Geometry: final body of the model. Coordinates: model frame, mm. Give positions to 0.01 mm unless a question says otherwise; leave off trailing zeros. Loops run counter-clockwise (first coordinate to the right, second up) from the corner with the lowest first, then second, coordinate; pieces in that order, holes last. Notation, with made-up numbers: (27.5, 70.5) - (37.5, 70.5) arc R24 ccw to (37.5, 108.5) - close; hole circle Ø5 at (7, 41). An arc over 180 degrees is marked (long way). Use one line per item in the form item = value.
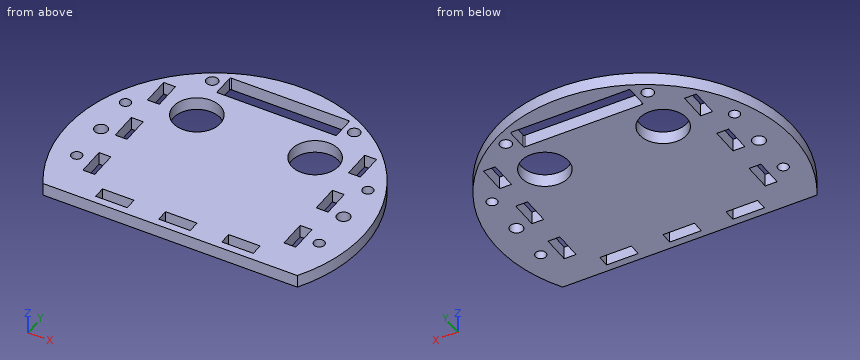
```python
from build123d import *

# Parameters (mm, degrees)
SKETCH1_R           = 2.25
SKETCH1_R_2         = 2.75
SKETCH1_R_3         = 2.5
SKETCH1_R_4         = 10
SKETCH1_W           = 13.333333333
SKETCH1_H           = 4.9958
SKETCH1_W_2         = 4.9958
SKETCH1_H_2         = 11.818181818
SKETCH1_H_3         = 11.818181819
SKETCH1_W_3         = 13.333333334
BOSS_EXTRUDE1_DEPTH = 5.4356


with BuildPart() as part:
    # Sketch1 → Boss-Extrude1 (new body)
    with BuildSketch(Plane.XY):
        with BuildLine():
            Line((-53.750203106, -32.862070326), (53.750203106, -32.862070326))
            ThreePointArc((53.750203106, -32.862070326), (0, 63), (-53.750203106, -32.862070326))
        make_face()
        with Locations((51.25, 23.184046239)):
            Circle(SKETCH1_R, mode=Mode.SUBTRACT)
        with Locations((51.25, -12.496398734)):
            Circle(SKETCH1_R, mode=Mode.SUBTRACT)
        with Locations((-51.25, -12.496398734)):
            Circle(SKETCH1_R, mode=Mode.SUBTRACT)
        with Locations((-51.25, 23.184046239)):
            Circle(SKETCH1_R, mode=Mode.SUBTRACT)
        with Locations((-51.25, 5.343823752)):
            Circle(SKETCH1_R_2, mode=Mode.SUBTRACT)
        with Locations((51.25, 5.343823752)):
            Circle(SKETCH1_R_2, mode=Mode.SUBTRACT)
        with Locations((-30.011103704, 49.928449687)):
            Circle(SKETCH1_R_3, mode=Mode.SUBTRACT)
        with Locations((30.011103704, 49.928449687)):
            Circle(SKETCH1_R_3, mode=Mode.SUBTRACT)
        with Locations((-25, 29.983449687)):
            Circle(SKETCH1_R_4, mode=Mode.SUBTRACT)
        with Locations((25, 29.983449687)):
            Circle(SKETCH1_R_4, mode=Mode.SUBTRACT)
        with BuildLine():
            Line((-24.765, 54.873449687), (24.765, 54.873449687))
            ThreePointArc((24.765, 54.873449687), (25.118553391, 54.727003078), (25.265, 54.373449687))
            Line((25.265, 54.373449687), (25.265, 45.483449687))
            ThreePointArc((25.265, 45.483449687), (25.118553391, 45.129896297), (24.765, 44.983449687))
            Line((24.765, 44.983449687), (-24.765, 44.983449687))
            ThreePointArc((-24.765, 44.983449687), (-25.118553391, 45.129896297), (-25.265, 45.483449687))
            Line((-25.265, 45.483449687), (-25.265, 54.373449687))
            ThreePointArc((-25.265, 54.373449687), (-25.118553391, 54.727003078), (-24.765, 54.873449687))
        make_face(mode=Mode.SUBTRACT)
        with Locations((-26.666666666, -27.189170326)):
            Rectangle(SKETCH1_W, SKETCH1_H, mode=Mode.SUBTRACT)
        with Locations((42.4979, 34.399638765)):
            Rectangle(SKETCH1_W_2, SKETCH1_H_2, mode=Mode.SUBTRACT)
        with Locations((42.4979, 10.763275129)):
            Rectangle(SKETCH1_W_2, SKETCH1_H_3, mode=Mode.SUBTRACT)
        with Locations((-42.4979, 34.399638765)):
            Rectangle(SKETCH1_W_2, SKETCH1_H_2, mode=Mode.SUBTRACT)
        with Locations((-42.4979, 10.763275129)):
            Rectangle(SKETCH1_W_2, SKETCH1_H_3, mode=Mode.SUBTRACT)
        with Locations((-42.4979, -12.873088508)):
            Rectangle(SKETCH1_W_2, SKETCH1_H_2, mode=Mode.SUBTRACT)
        with Locations((42.4979, -12.873088508)):
            Rectangle(SKETCH1_W_2, SKETCH1_H_2, mode=Mode.SUBTRACT)
        with Locations((0, -27.189170326)):
            Rectangle(SKETCH1_W_3, SKETCH1_H, mode=Mode.SUBTRACT)
        with Locations((26.666666666, -27.189170326)):
            Rectangle(SKETCH1_W, SKETCH1_H, mode=Mode.SUBTRACT)
    extrude(amount=BOSS_EXTRUDE1_DEPTH)


solid = part.part
```
(1) Cut plane C-C (y = 13). Return the cut outline in (x, z), plus the area to 3 significant figures.
Solution:
outline = (-61.64, 0) - (-45, 0) - (-45, 5.44) - (-61.64, 5.44) - close; (-40, 0) - (40, 0) - (40, 5.44) - (-40, 5.44) - close; (45, 0) - (61.64, 0) - (61.64, 5.44) - (45, 5.44) - close
area = 616 mm2
(2) Material intervals for L1, parallel to Y at x = -51.25, z = 2.6; L2, parallel to Y at x = -5.5, z = 2.1; L3, parallel to Y at x = -25, z = 3.15, sorted ascending. Write a range as from..to.
Solution:
L1 = -32.86..-14.75, -10.25..2.59, 8.09..20.93, 25.43..36.64
L2 = -32.86..-29.69, -24.69..44.98, 54.87..62.76
L3 = -32.86..-29.69, -24.69..19.98, 39.98..45.04, 54.81..57.83
(3) Cut plane B-B (x = 51.25). Return the cut outline in (y, z).
Solution:
outline = (-32.86, 0) - (-14.75, 0) - (-14.75, 5.44) - (-32.86, 5.44) - close; (-10.25, 0) - (2.59, 0) - (2.59, 5.44) - (-10.25, 5.44) - close; (8.09, 0) - (20.93, 0) - (20.93, 5.44) - (8.09, 5.44) - close; (25.43, 0) - (36.64, 0) - (36.64, 5.44) - (25.43, 5.44) - close
(4) Cut plane A-A (x = 0). Return the cut outline in (y, z), plus the area to 3 significant figures.
Solution:
outline = (-32.86, 0) - (-29.69, 0) - (-29.69, 5.44) - (-32.86, 5.44) - close; (-24.69, 0) - (44.98, 0) - (44.98, 5.44) - (-24.69, 5.44) - close; (54.87, 0) - (63, 0) - (63, 5.44) - (54.87, 5.44) - close
area = 440 mm2
(5) Pin query (flat end, axial travel): P1, Ø1, axis at y = 32, z = 4, coming from the +X side; P2, Ø1.5, axis at y = -26.5, z = 4, coming from the +X side; P3, Ø1.6, axis at y = 8.5, z = 1.5, coming from the +X side. Return the tip coordinate at first contact, or that it passes through.
Solution:
P1 = 54.56
P2 = 57.5
P3 = 62.53
(6) Cut plane D-D (z = 1.9). Give the number of separate pieces and of enclosed holes in the cut face, plus the area to 3 significant figures.
Solution:
separate_pieces = 1
enclosed_holes = 20
area = 8,350 mm2
